Autodesk Inventor part; units mm, degrees
ref_plane "YZ Plane" through (0, 0, 0) normal (1, 0, 0) x (0, 1, 0)
ref_plane "XZ Plane" through (0, 0, 0) normal (0, 1, 0) x (-1, 0, 0)
ref_plane "XY Plane" through (0, 0, 0) normal (0, 0, 1) x (1, 0, 0)
sketch "Sketch1" plane through (0, 0, 0) normal (0, 1, 0) x (-1, 0, 0)
  circle A0 centre (0, 0) radius 16.575
  dimension "d0" = 33.15
extrude "Extrusion1" add sketch "Sketch1" along normal blind 3.8
sketch "Sketch2" plane through (0, 3.8, 0) normal (0, 1, 0) x (1, 0, 0)
  circle A0 centre (0, 0) radius 16.575
  circle A1 centre (0, 0) radius 14
  dimension "d3" = 28
extrude "Extrusion2" add sketch "Sketch2" along normal blind 1 contours A1
sketch "Sketch3" plane through (0, 4.8, 0) normal (0, 1, 0) x (1, 0, 0)
  circle A0 centre (0, 0) radius 14
  circle A1 centre (0, 0) radius 5
  dimension "d6" = 10
extrude "Extrusion3" add sketch "Sketch3" along normal blind 3.8 contours A1
sketch "Sketch4" plane through (0, 8.6, 0) normal (0, 1, 0) x (1, 0, 0)
  circle A0 centre (0, 0) radius 5
  circle A1 centre (0, 0) radius 1.8
  dimension "d9" = 3.6
extrude "Extrusion4" cut sketch "Sketch4" against normal blind 3.6 contours A1
sketch "Sketch5" plane through (0, 8.6, 0) normal (0, 1, 0) x (1, 0, 0)
  circle A0 centre (0, 0) radius 1.8
  circle A1 centre (0, 0) radius 5
  circle A2 centre (0, 0) radius 3
  dimension "d12" = 6
extrude "Extrusion5" cut sketch "Sketch5" against normal blind 3.6 contours A2
sketch "Sketch6" plane through (0, 0, 0) normal (0, -1, 0) x (1, 0, 0)
  circle A0 centre (0, 0) radius 16.575
  circle A1 centre (0, 0) radius 3
  dimension "d15" = 6
extrude "Extrusion6" cut sketch "Sketch6" against normal blind 3.8 contours A1
properties part number "kolecko_servo(3)"
CAD build for the part. Positions are in the model's coordinates, mm. A direction names the side the tool comes from. Round coordinates to 2 decimals unless told otherwise and drop trailing zeros. Order: outer loops, then holes, each group sorted by start corner. A loop starts at its lowest first (then second) coordinate and runs counter-clockwise, first axis right, second up. Notation, with made-up numbers: (-13.75, -7) - (17.25, -7) arc R25 ccw to (17.25, 17) - close; hole circle Ø4 at (-34.75, 37). An arc over 180 degrees is marked (long way). Answer in a Markdown table with one row per item. Add a question column.
(1) 3-axis set-ups, long thin cutter, end or side, ignore diameter. For faces 4 (the face through (3.59, 1.87, 16.18)), 5 (the face through (0, 5, 0)), 6 (the face through (0, 3.8, 0)): which of +Z, -Z, +X, -X, +Y, -Y reach the whole face in a straight line?
(2) Probe L1, parallel to Z at x = 0, y = 6.4; L2, parallel to X at y = 6.25, z = -4. List the from-to ranges inside material, lowest first. Write a range as [from, to].
(3) Band-saw the part on C-C on y = 1.75. List the corners of the cut face in (x, z) (3 decimals).
(4) Band-saw the part on D-D on z = -11. List the corners of the cut face in (x, y).
(5) Band-saw the part on A-A on x = 0. List the corners of the cut face in (y, z) (3 decimals).
(6) Drop flat-ended pins along their axis: pin 1 Ø5 at (y, z) = (1, 7.5) entering from +X; pin 2 Ø3 at (x, z) = (-3.5, 8) entering from +Y; pin 3 Ø3.5 at (x, z) = (0, 0) entering from -Y. Give the stop position or say it passes through.
(7) Band-saw the part on B-B on z = 0. List the corners of the cut face in (x, y) (3 decimals), and give its area (3 significant figures).
(8) Mould opens along Z. For faces 1 (the face through (12.932, 4.293, -5.362)), 2 (the face through (3.3, 8.6, -0.1)), 3 (the face through (-3, 7, 0)) say: +Z half, -Z half, draft (parallel to the pull), parting line (faces both ways), or undercut.
Data:
| question | item | result |
|---|---|---|
| 1 | face 4 | +Y, -Y |
| 1 | face 5 | +Y |
| 1 | face 6 | -Y |
| 2 | L1 | z = [-5, -3], [3, 5] |
| 2 | L2 | x = [-3, 3] |
| 3 | outline | circle Ø33.15 at (0, 0); hole circle Ø6 at (0, 0) |
| 4 | outline | (-12.4, 0) - (12.4, 0) - (12.4, 3.8) - (8.66, 3.8) - (8.66, 4.8) - (-8.66, 4.8) - (-8.66, 3.8) - (-12.4, 3.8) - close |
| 5 | outline | (0, -16.575) - (3.8, -16.575) - (3.8, -14) - (4.8, -14) - (4.8, -5) - (8.6, -5) - (8.6, -3) - (5, -3) - (5, 3) - (8.6, 3) - (8.6, 5) - (4.8, 5) - (4.8, 14) - (3.8, 14) - (3.8, 16.575) - (0, 16.575) - (0, 3) - (3.8, 3) - (3.8, -3) - (0, -3) - close |
| 6 | pin 1 | stops at x = 15.8 |
| 6 | pin 2 | stops at y = 4.8 |
| 6 | pin 3 | stops at y = 3.8 |
| 7 | outline | (-16.575, 0) - (-3, 0) - (-3, 3.8) - (3, 3.8) - (3, 0) - (16.575, 0) - (16.575, 3.8) - (14, 3.8) - (14, 4.8) - (5, 4.8) - (5, 8.6) - (3, 8.6) - (3, 5) - (-3, 5) - (-3, 8.6) - (-5, 8.6) - (-5, 4.8) - (-14, 4.8) - (-14, 3.8) - (-16.575, 3.8) - close |
| 7 | area | 148 mm^2 |
| 8 | face 1 | parting line |
| 8 | face 2 | draft |
| 8 | face 3 | undercut |
